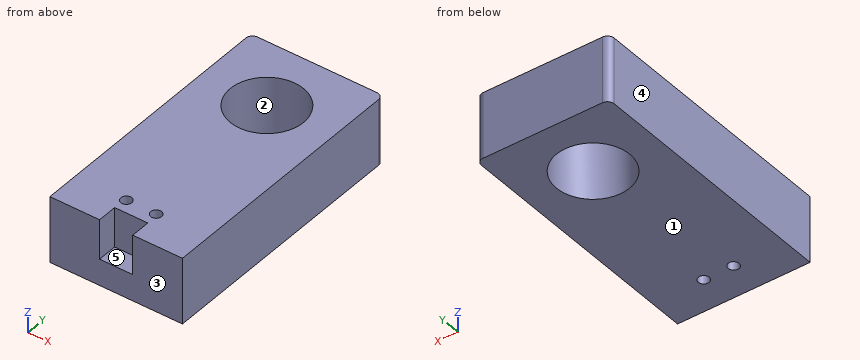
```python
from build123d import *

# Parameters (mm, degrees)
SKETCH_1_W          = 40
SKETCH_1_H          = 40
EXTRUDE_1_DEPTH     = 20
SKETCH_2_R          = 11.05
CUT_EXTRUDE_1_DEPTH = 20
SKETCH_3_W          = 40
SKETCH_3_H          = 20
EXTRUDE_2_DEPTH     = 40
SKETCH_4_R          = 1.65
CUT_EXTRUDE_2_DEPTH = 40
SKETCH_5_W          = 10
SKETCH_5_H          = 12
CUT_EXTRUDE_3_DEPTH = 6
FILLET_1_R          = 2


with BuildPart() as part:
    # 草图1 → 凸台-拉伸1 (new body)
    with BuildSketch(Plane.XY):
        Rectangle(SKETCH_1_W, SKETCH_1_H)
    extrude(amount=EXTRUDE_1_DEPTH)

    # 草图2 → 切除-拉伸1 (cut)
    with BuildSketch(Plane.XY.offset(20)):
        Circle(SKETCH_2_R)
    extrude(amount=-CUT_EXTRUDE_1_DEPTH, mode=Mode.SUBTRACT)

    # 草图3 → 凸台-拉伸2 (add)
    with BuildSketch(Plane.XZ.offset(20)):
        with Locations((0, 10)):
            Rectangle(SKETCH_3_W, SKETCH_3_H)
    extrude(amount=EXTRUDE_2_DEPTH)

    # 草图4 → 切除-拉伸2 (cut)
    with BuildSketch(Plane.XY.offset(20)):
        with Locations((4.5, -50)):
            Circle(SKETCH_4_R)
        with Locations((-4.5, -50)):
            Circle(SKETCH_4_R)
    extrude(amount=-CUT_EXTRUDE_2_DEPTH, mode=Mode.SUBTRACT)

    # 草图5 → 切除-拉伸3 (cut)
    with BuildSketch(Plane.XZ.offset(60)):
        with Locations((0, 14)):
            Rectangle(SKETCH_5_W, SKETCH_5_H)
    extrude(amount=-CUT_EXTRUDE_3_DEPTH, mode=Mode.SUBTRACT)

    # 圆角1
    fillet_1_edges = [part.edges().sort_by_distance(p)[0] for p in [
        (-20, 20, 10),
        (20, 20, 10),
    ]]
    fillet(fillet_1_edges, radius=FILLET_1_R)


solid = part.part
```
Source: CAD feature listing. Evaluate the final solid. Frame: model axes, mm. Face numbers are marked on the shaded views. A direction names the side the tool comes from. Coordinates: 2 decimals unless noted, no trailing zeros. Write each loop counter-clockwise with the first axis right and the second up, starting at its lowest first coordinate (ties: lowest second). Pieces come first, ordered by that corner, then holes. Notation, with made-up numbers: (82.25, -33.75) -> (126.25, -33.75) arc R34 ccw to (126.25, 5.25) -> close; hole circle Ø8 at (-37.5, 34.25). An arc over 180 degrees is marked (long way). Return JSON: item names as keys, results as strings. Group by question number.
1) Mould query, pull axis Y, two halves, no side actions, for the marked faces 1, 2 and 3. Classes: +Y half, -Y half, draft (parallel to the pull), parting line (faces both ways), or undercut.
2) Ray query, line 1 along Y through (x, z) = (0.5, 9.5); line 2 along Y through (x, z) = (0, 6); line 3 along Y through (x, z) = (5.5, 12.25). Return the intervals inside material, ascending.
3) Section query D-D, the plane x = -10. Return loops of the section in (y, z), plus the area to 3 significant figures.
4) Contact query for flat-ended pins moving along their axis: P1, Ø5, axis at x = 0.5, y = -58.5, coming from the +Z side; P2, Ø4, axis at x = 4.5, y = -50, coming from the -Z side; P3, Ø6, axis at x = -0.5, z = 16, coming from the -Y side; P4, Ø13.5, axis at x = 0, y = 0, coming from the -Z side. Output: stop coordinate, or through.
5) Section query C-C, the plane z = 13.75. Return loops of the section in (x, y), plus the area to 3 significant figures.
6) Set-up query: the marked faces 4 and 5. Return all of +Z, -Z, +X, -X, +Y, -Y with unobstructed straight access to the full face (end or side cutting, diameter ignored); none if empty.
7) Section query A-A, the plane y = -50. Return loops of the section in (x, z), plus the area to 3 significant figures.
8) Section query B-B, the plane y = 0. Return loops of the section in (x, z), plus the area to 3 significant figures.
From the geometry:
{
 "1": {"face 1": "draft", "face 2": "undercut", "face 3": "-Y half"},
 "2": {"line 1": "-54 to -11.04, 11.04 to 20", "line 2": "-60 to -11.05, 11.05 to 20", "line 3": "-60 to -51.31, -48.69 to -9.58, 9.58 to 20"},
 "3": {"outline": "(-60, 0) -> (-4.7, 0) -> (-4.7, 20) -> (-60, 20) -> close; (4.7, 0) -> (20, 0) -> (20, 20) -> (4.7, 20) -> close", "area": "1,410 mm²"},
 "4": {"P1": "z = 8", "P2": "z = 0", "P3": "y = -54", "P4": "through"},
 "5": {"outline": "(-20, -60) -> (-5, -60) -> (-5, -54) -> (5, -54) -> (5, -60) -> (20, -60) -> (20, 18) arc R2 ccw to (18, 20) -> (-18, 20) arc R2 ccw to (-20, 18) -> close; hole circle Ø22.1 at (0, 0); hole circle Ø3.3 at (-4.5, -50); hole circle Ø3.3 at (4.5, -50)", "area": "2,740 mm²"},
 "6": {"face 4": "+Z, -Z, -X, +Y, -Y", "face 5": "+Z, -Y"},
 "7": {"outline": "(-20, 0) -> (-6.15, 0) -> (-6.15, 20) -> (-20, 20) -> close; (-2.85, 0) -> (2.85, 0) -> (2.85, 20) -> (-2.85, 20) -> close; (6.15, 0) -> (20, 0) -> (20, 20) -> (6.15, 20) -> close", "area": "668 mm²"},
 "8": {"outline": "(-20, 0) -> (-11.05, 0) -> (-11.05, 20) -> (-20, 20) -> close; (11.05, 0) -> (20, 0) -> (20, 20) -> (11.05, 20) -> close", "area": "358 mm²"}
}
